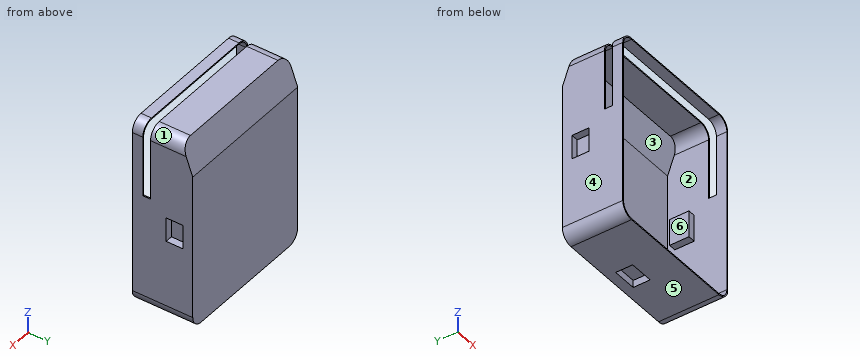
```python
from build123d import *

# Parameters (mm, degrees)
BOSS_EXTRUDE1_DEPTH     = 200
BOSS_EXTRUDE2_DEPTH     = 50
DRAFT2_START            = 200
DRAFT2_DEPTH            = 50
DRAFT2_START_2          = 192.170637281
DRAFT2_2_OUTLINE_W      = 602
DRAFT2_2_OUTLINE_H      = 136
DRAFT2_2_DEPTH          = 43.829362719
SKETCH12_W              = 100
SKETCH12_H              = 70
CUT_EXTRUDE4_DEPTH      = 30
SKETCH14_W              = 100
SKETCH14_H              = 70
CUT_EXTRUDE5_DEPTH      = 30
SKETCH13_W              = 100
SKETCH13_H              = 70
CUT_EXTRUDE2_DEPTH      = 30
SHELL1_T                = -5
CUT_EXTRUDE6_DEPTH      = 1012.496416207
CUT_EXTRUDE6_DEPTH_BACK = 1012.496416207
SKETCH15_W              = 300
SKETCH15_H              = 32


with BuildPart() as part:
    # Sketch1 → Boss-Extrude1 (new body)
    with BuildSketch(Plane(origin=(0, 0, 0), x_dir=(1, 0, 0), z_dir=(0, 1, 0))):
        with BuildLine():
            Line((50, 0), (550, 0))
            ThreePointArc((550, 0), (585.355339059, 14.644660941), (600, 50))
            Line((600, 50), (600, 725))
            ThreePointArc((600, 725), (585.355339059, 760.355339059), (550, 775))
            Line((550, 775), (50, 775))
            ThreePointArc((50, 775), (14.644660941, 760.355339059), (0, 725))
            Line((0, 725), (0, 50))
            ThreePointArc((0, 50), (14.644660941, 14.644660941), (50, 0))
        make_face()
    extrude(amount=BOSS_EXTRUDE1_DEPTH)

    # Sketch5 → Boss-Extrude2 (add)
    with BuildSketch(Plane(origin=(0, 200, 0), x_dir=(1, 0, 0), z_dir=(0, 1, 0))):
        with BuildLine():
            Line((600, 125), (0, 125))
            Line((0, 125), (0, 725))
            ThreePointArc((0, 725), (14.644660941, 760.355339059), (50, 775))
            Line((50, 775), (550, 775))
            ThreePointArc((550, 775), (585.355339059, 760.355339059), (600, 725))
            Line((600, 725), (600, 125))
        make_face()
    extrude(amount=BOSS_EXTRUDE2_DEPTH)

    # Draft2: read off the stored shape, not the designer's step
    # Draft2 outline → Draft2 (add)
    with BuildSketch(Plane(origin=(0, 0, 0), x_dir=(1, 0, 0), z_dir=(0, 1, 0)).offset(DRAFT2_START)):
        with BuildLine():
            ThreePointArc((550, 0), (585.355339059, 14.644660941), (600, 50))
            Line((600, 50), (600, 125))
            Line((600, 125), (0, 125))
            Line((0, 125), (0, 50))
            ThreePointArc((0, 50), (14.644660941, 14.644660941), (50, 0))
            Line((50, 0), (550, 0))
        make_face()
    extrude(amount=DRAFT2_DEPTH)

    # Draft2 2 outline → Draft2 2 (cut)
    with BuildSketch(Plane(origin=(0, 0, 0), x_dir=(1, 0, 0), z_dir=(0, 0.9396926207859094, 0.34202014332566616)).offset(DRAFT2_START_2)):
        with Locations((300, 136)):
            Rectangle(DRAFT2_2_OUTLINE_W, DRAFT2_2_OUTLINE_H)
    extrude(amount=DRAFT2_2_DEPTH, mode=Mode.SUBTRACT)

    # Sketch12 → Cut-Extrude4 (cut)
    with BuildSketch(Plane(origin=(0, 0, 0), x_dir=(0, 0, -1), z_dir=(1, 0, 0))):
        with Locations((400, 175)):
            Rectangle(SKETCH12_W, SKETCH12_H)
    extrude(amount=CUT_EXTRUDE4_DEPTH, mode=Mode.SUBTRACT)

    # Sketch14 → Cut-Extrude5 (cut)
    with BuildSketch(Plane(origin=(600, 0, 0), x_dir=(0, 0, -1), z_dir=(1, 0, 0))):
        with Locations((400, 175)):
            Rectangle(SKETCH14_W, SKETCH14_H)
    extrude(amount=-CUT_EXTRUDE5_DEPTH, mode=Mode.SUBTRACT)

    # Sketch13 → Cut-Extrude2 (cut)
    with BuildSketch(Plane(origin=(0, 0, -775), x_dir=(-1, 0, 0), z_dir=(0, 0, -1))):
        with Locations((-300, 175)):
            Rectangle(SKETCH13_W, SKETCH13_H)
    extrude(amount=-CUT_EXTRUDE2_DEPTH, mode=Mode.SUBTRACT)

    # Shell1
    shell1_openings = [part.faces().sort_by_distance(p)[0] for p in [
        (300, 0, -387.5),
    ]]
    offset(amount=SHELL1_T, openings=shell1_openings, kind=Kind.INTERSECTION)

    # Sketch15 → Cut-Extrude6 (cut, two sides: drawn at the far end of the back side and taken through both)
    with BuildSketch(Plane.ZY.offset(-CUT_EXTRUDE6_DEPTH_BACK)):
        with Locations((-150, 59.4)):
            Rectangle(SKETCH15_W, SKETCH15_H)
    extrude(amount=CUT_EXTRUDE6_DEPTH + CUT_EXTRUDE6_DEPTH_BACK, mode=Mode.SUBTRACT)


solid = part.part
```
Input: part model. Units: mm. Frame: model coordinates. Face numbers are marked on the shaded views. A direction names the side the tool comes from. Give positions to 0.01 mm unless a question says otherwise; leave off trailing zeros. Order: outer loops, then holes, each group sorted by start corner. A loop starts at its lowest first (then second) coordinate and runs counter-clockwise, first axis right, second up.
1. Draft query along X for the marked faces 1, 2, 3 and 4. Return one class per face: released by +X, released by -X, zero draft, split by the parting line, or undercut.
Computed:
face 1: released by +X
face 2: undercut
face 3: undercut
face 4: released by -X
2. Line query: probe 1 along X at (y, z) = (64, -537.5); probe 2 along Z at (x, y) = (458, 16.5); probe 3 along Z at (x, y) = (297.5, 157). Output: solid intervals per line, ascending.
Computed:
probe 1: x = 0 to 5, 595 to 600
probe 2: z = -775 to -770, -5 to 0
probe 3: z = -745 to -740, -5 to 0
3. Cut plane C-C (z = -415). Return loops of the section in (x, y).
Computed:
outline: (0, 0) - (5, 0) - (5, 135) - (35, 135) - (35, 215) - (5, 215) - (5, 245) - (595, 245) - (595, 215) - (565, 215) - (565, 135) - (595, 135) - (595, 0) - (600, 0) - (600, 140) - (570, 140) - (570, 210) - (600, 210) - (600, 250) - (0, 250) - (0, 210) - (30, 210) - (30, 140) - (0, 140) - close
4. Cut plane D-D (y = 66.5). Return loops of the section in (x, z), and give its area (3 significant figures).
Computed:
outline: (0, -725) arc R50 ccw to (50, -775) - (550, -775) arc R50 ccw to (600, -725) - (600, -300) - (595, -300) - (595, -725) arc R45 cw to (550, -770) - (50, -770) arc R45 cw to (5, -725) - (5, -300) - (0, -300) - close
area: 7,500 mm2
5. Set-up query: the marked faces 5 and 6. Return all of +Z, -Z, +X, -X, +Y, -Y with unobstructed straight access to the full face (end or side cutting, diameter ignored); none if empty.
Computed:
face 5: -Z, +X, -X, +Y, -Y
face 6: -Y
6. Pin query (flat end, axial travel): pin 1 Ø2 at (x, y) = (453.5, 60.5) entering from +Z; pin 2 Ø9 at (x, z) = (7.5, -392.5) entering from -Y; pin 3 Ø9 at (x, y) = (13.5, 168.5) entering from -Z; pin 4 Ø24 at (y, z) = (193, -762) entering from +X. Return the tip coordinate at first contact, or that it passes through.
Computed:
pin 1: stops at z = -770
pin 2: stops at y = 0
pin 3: stops at z = -763.42
pin 4: stops at x = 593.3
7. Cut plane A-A (x = 171.5). Return loops of the section in (y, z), and give its area (3 significant figures).
Computed:
outline: (0, -775) - (250, -775) - (250, -125) - (204.5, 0) - (75.4, 0) - (75.4, -5) - (201, -5) - (245, -125.88) - (245, -770) - (0, -770) - close; (0, -5) - (43.4, -5) - (43.4, 0) - (0, 0) - close
area: 5,980 mm2
8. Cut plane B-B (z = -170.5). Return loops of the section in (x, y).
Computed:
outline: (0, 0) - (5, 0) - (5, 43.4) - (0, 43.4) - close; (0, 75.4) - (5, 75.4) - (5, 245) - (595, 245) - (595, 75.4) - (600, 75.4) - (600, 250) - (0, 250) - close; (595, 0) - (600, 0) - (600, 43.4) - (595, 43.4) - close
